Here's how the part is built. I have some questions about the finished solid (model axes, mm). Coordinates: 2 decimals unless noted, no trailing zeros. Loops run counter-clockwise (first coordinate to the right, second up) from the corner with the lowest first, then second, coordinate; pieces in that order, holes last. Notation, with made-up numbers: (-12.75, 64.5) - (36.25, 64.5) arc R19 cw to (36.25, 68.5) - close; hole circle Ø1 at (-27.75, 48). An arc over 180 degrees is marked (long way). Use a Markdown table: item, result.
```python
from build123d import *

# Parameters (mm, degrees)
EXTRUDE_1_DEPTH                  = 345
HOLE_WIZARD_M6_78051_D           = 6
HOLE_WIZARD_M6_78051_CBORE_D     = 9.5
HOLE_WIZARD_M6_78051_CBORE_DEPTH = 8.5
PATTERN_LINEAR_1_COUNT           = 6
PATTERN_LINEAR_1_PITCH           = 60
PATTERN_LINEAR_2_COUNT           = 6
PATTERN_LINEAR_2_PITCH           = 60


with BuildPart() as part:
    # Эскиз1 → Бобышка-Вытянуть1 (new, symmetric)
    with BuildSketch(Plane(origin=(0, 0, 0), x_dir=(0, 0, -1), z_dir=(1, 0, 0))):
        with BuildLine():
            Line((-10, 0.989949494), (-9.010050506, 0))
            Line((-9.010050506, 0), (9.010050506, 0))
            Line((9.010050506, 0), (10, 0.989949494))
            Line((10, 0.989949494), (10, 4))
            Line((10, 4), (6.6, 7.4))
            Line((6.6, 7.4), (6.6, 9.9))
            Line((6.6, 9.9), (7.5, 10.8))
            ThreePointArc((7.5, 10.8), (8.173654403, 12.426345597), (9.8, 13.1))
            Line((9.8, 13.1), (10, 13.3))
            Line((10, 13.3), (10, 14.9))
            Line((10, 14.9), (9.8, 15.1))
            ThreePointArc((9.8, 15.1), (8.173654403, 15.773654403), (7.5, 17.4))
            Line((7.5, 17.4), (7.4, 17.5))
            Line((7.4, 17.5), (-7.4, 17.5))
            Line((-7.4, 17.5), (-7.5, 17.4))
            ThreePointArc((-7.5, 17.4), (-8.173654403, 15.773654403), (-9.8, 15.1))
            Line((-9.8, 15.1), (-10, 14.9))
            Line((-10, 14.9), (-10, 13.3))
            Line((-10, 13.3), (-9.8, 13.1))
            ThreePointArc((-9.8, 13.1), (-8.173654403, 12.426345597), (-7.5, 10.8))
            Line((-7.5, 10.8), (-6.6, 9.9))
            Line((-6.6, 9.9), (-6.6, 7.4))
            Line((-6.6, 7.4), (-10, 4))
            Line((-10, 4), (-10, 0.989949494))
        make_face()
    extrude(amount=EXTRUDE_1_DEPTH, both=True)

    # Цековка M6 для болта с шестигранной головкой класса А ГОСТ 78051 (through all)
    with Locations(Plane.ZX.offset(17.5)):
        with Locations((0, 0)):
            hole_wizard_m6_78051 = CounterBoreHole(HOLE_WIZARD_M6_78051_D / 2, HOLE_WIZARD_M6_78051_CBORE_D / 2, HOLE_WIZARD_M6_78051_CBORE_DEPTH)

    # Линейный массив1: Цековка M6 для болта с шестигранной головкой класса А ГОСТ 78051 ×6
    with Locations(*[(i * PATTERN_LINEAR_1_PITCH, 0, 0) for i in range(1, PATTERN_LINEAR_1_COUNT)]):
        add(hole_wizard_m6_78051, mode=Mode.SUBTRACT)

    # Линейный массив2: Цековка M6 для болта с шестигранной головкой класса А ГОСТ 78051 ×6
    with Locations(*[(-i * PATTERN_LINEAR_2_PITCH, 0, 0) for i in range(1, PATTERN_LINEAR_2_COUNT)]):
        add(hole_wizard_m6_78051, mode=Mode.SUBTRACT)


solid = part.part
```
Q1. Will these pins go through, and if not, where does the flat tip stop? P1, Ø7, axis at x = -60, z = 0, coming from the -Y side; P2, Ø3, axis at x = -302, z = -1.5, coming from the +Y side; P3, Ø3, axis at x = -127, y = 6, coming from the +Z side; P4, Ø3, axis at x = -29, y = 9, coming from the +Z side.
Check values:
| item | result |
|---|---|
| P1 | y = 0 |
| P2 | y = 9 |
| P3 | z = 9.5 |
| P4 | z = 7.2 |
Q2. I want a section at A-A, the plane x = -278. Write out the boundary of the cut face in (y, z), then the cut area to 3 significant figures.
Check values:
| item | result |
|---|---|
| outline | (0, -9.01) - (0.99, -10) - (4, -10) - (7.4, -6.6) - (9.9, -6.6) - (10.8, -7.5) arc R2.3 cw to (13.1, -9.8) - (13.3, -10) - (14.9, -10) - (15.1, -9.8) arc R2.3 cw to (17.4, -7.5) - (17.5, -7.4) - (17.5, 7.4) - (17.4, 7.5) arc R2.3 cw to (15.1, 9.8) - (14.9, 10) - (13.3, 10) - (13.1, 9.8) arc R2.3 cw to (10.8, 7.5) - (9.9, 6.6) - (7.4, 6.6) - (4, 10) - (0.99, 10) - (0, 9.01) - close |
| area | 296 mm^2 |
Q3. Please list where these lines run through material, in increasing order: L1, parallel to Z at x = 300, y = 4; L2, parallel to Z at x = 119, y = 11.5; L3, parallel to Z at x = -161.5, y = 9.75. Write a range as from..to.
Check values:
| item | result |
|---|---|
| L1 | -10..-3, 3..10 |
| L2 | -7.61..-4.64, 4.64..7.61 |
| L3 | -6.6..6.6 |
